Design review of the part built by this model. Coordinates are the model's own, in mm. Give positions to 0.01 mm unless a question says otherwise; leave off trailing zeros. Order: outer loops, then holes, each group sorted by start corner. A loop starts at its lowest first (then second) coordinate and runs counter-clockwise, first axis right, second up. Notation, with made-up numbers: M -23,21.5 L 14,21.5 A15 cw 14,47.5 Z; hole C 48.5,68.5 d7. An arc over 180 degrees is marked long. Answer as a JSON object with one key per item and string values.
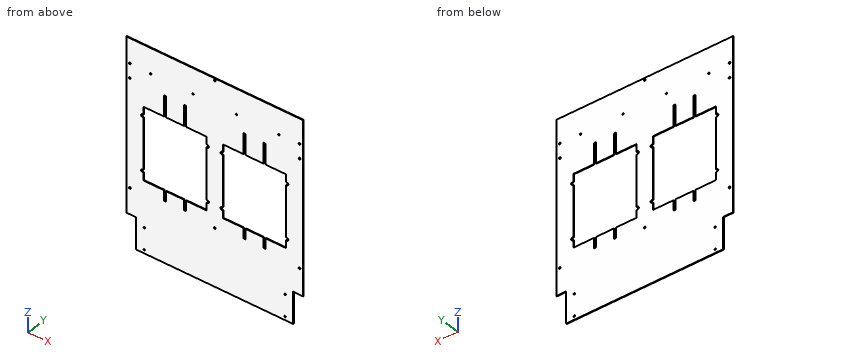
from build123d import *

# Parameters (mm, degrees)
F0_W     = 622.3
F0_H     = 717.55
F0_R     = 2.579688
F0_R_2   = 3.175
F1_DEPTH = 1.27
F2_W     = 34.925
F2_H     = 111.125
F2_W_2   = 6.35
F2_H_2   = 73.025
F2_H_3   = 36.5125
F2_R     = 2.579688
F3_DEPTH = 2.541


with BuildPart() as f1:
    # F0 (on Front) → F1 (new body, symmetric)
    with BuildSketch(Plane.XZ):
        Rectangle(F0_W, F0_H)
        with Locations((-247.65, -346.075)):
            Circle(F0_R, mode=Mode.SUBTRACT)
        with Locations((-247.65, -269.875)):
            Circle(F0_R, mode=Mode.SUBTRACT)
        with Locations((-298.45, -156.718)):
            Circle(F0_R_2, mode=Mode.SUBTRACT)
        with Locations((247.65, -346.075)):
            Circle(F0_R, mode=Mode.SUBTRACT)
        with Locations((247.65, -269.875)):
            Circle(F0_R, mode=Mode.SUBTRACT)
        with Locations((0, -156.718)):
            Circle(F0_R_2, mode=Mode.SUBTRACT)
        with Locations((298.45, -156.718)):
            Circle(F0_R_2, mode=Mode.SUBTRACT)
        with BuildLine():
            Line((-250.825, 117.856), (-250.825, 144.78))
            Line((-250.825, 144.78), (-28.575, 144.78))
            Line((-28.575, 144.78), (-28.575, 117.856))
            Line((-28.575, 117.856), (-25.4, 117.856))
            ThreePointArc((-25.4, 117.856), (-20.574, 113.03), (-25.4, 108.204))
            Line((-25.4, 108.204), (-28.575, 108.204))
            Line((-28.575, 108.204), (-28.575, -72.644))
            Line((-28.575, -72.644), (-25.4, -72.644))
            ThreePointArc((-25.4, -72.644), (-20.574, -77.47), (-25.4, -82.296))
            Line((-25.4, -82.296), (-28.575, -82.296))
            Line((-28.575, -82.296), (-28.575, -109.22))
            Line((-28.575, -109.22), (-250.825, -109.22))
            Line((-250.825, -109.22), (-250.825, -82.296))
            Line((-250.825, -82.296), (-254, -82.296))
            ThreePointArc((-254, -82.296), (-258.826, -77.47), (-254, -72.644))
            Line((-254, -72.644), (-250.825, -72.644))
            Line((-250.825, -72.644), (-250.825, 108.204))
            Line((-250.825, 108.204), (-254, 108.204))
            ThreePointArc((-254, 108.204), (-258.826, 113.03), (-254, 117.856))
            Line((-254, 117.856), (-250.825, 117.856))
        make_face(mode=Mode.SUBTRACT)
        with Locations((-298.45, 221.107)):
            Circle(F0_R_2, mode=Mode.SUBTRACT)
        with Locations((-298.45, 271.907)):
            Circle(F0_R_2, mode=Mode.SUBTRACT)
        with BuildLine():
            Line((28.575, -109.22), (28.575, -82.296))
            Line((28.575, -82.296), (25.4, -82.296))
            ThreePointArc((25.4, -82.296), (20.574, -77.47), (25.4, -72.644))
            Line((25.4, -72.644), (28.575, -72.644))
            Line((28.575, -72.644), (28.575, 108.204))
            Line((28.575, 108.204), (25.4, 108.204))
            ThreePointArc((25.4, 108.204), (20.574, 113.03), (25.4, 117.856))
            Line((25.4, 117.856), (28.575, 117.856))
            Line((28.575, 117.856), (28.575, 144.78))
            Line((28.575, 144.78), (250.825, 144.78))
            Line((250.825, 144.78), (250.825, 117.856))
            Line((250.825, 117.856), (254, 117.856))
            ThreePointArc((254, 117.856), (258.826, 113.03), (254, 108.204))
            Line((254, 108.204), (250.825, 108.204))
            Line((250.825, 108.204), (250.825, -72.644))
            Line((250.825, -72.644), (254, -72.644))
            ThreePointArc((254, -72.644), (258.826, -77.47), (254, -82.296))
            Line((254, -82.296), (250.825, -82.296))
            Line((250.825, -82.296), (250.825, -109.22))
            Line((250.825, -109.22), (28.575, -109.22))
        make_face(mode=Mode.SUBTRACT)
        with Locations((0, 351.282)):
            Circle(F0_R_2, mode=Mode.SUBTRACT)
        with Locations((298.45, 221.107)):
            Circle(F0_R_2, mode=Mode.SUBTRACT)
        with Locations((298.45, 271.907)):
            Circle(F0_R_2, mode=Mode.SUBTRACT)
    extrude(amount=F1_DEPTH, both=True)

    # F2 (on face) → F3 (cut, through all)
    with BuildSketch(Plane.XZ.offset(1.27)):
        with Locations((-293.6875, -303.2125)):
            Rectangle(F2_W, F2_H)
        with Locations((293.6875, -303.2125)):
            Rectangle(F2_W, F2_H)
        with Locations((-174.625, 181.2925)):
            Rectangle(F2_W_2, F2_H_2)
        with Locations((-104.775, 181.2925)):
            Rectangle(F2_W_2, F2_H_2)
        with Locations((-104.775, -127.47625)):
            Rectangle(F2_W_2, F2_H_3)
        with Locations((-174.625, -127.47625)):
            Rectangle(F2_W_2, F2_H_3)
        with Locations((104.775, 181.2925)):
            Rectangle(F2_W_2, F2_H_2)
        with Locations((174.625, -127.47625)):
            Rectangle(F2_W_2, F2_H_3)
        with Locations((174.625, 181.2925)):
            Rectangle(F2_W_2, F2_H_2)
        with Locations((104.775, -127.47625)):
            Rectangle(F2_W_2, F2_H_3)
        with Locations((225.425, 269.875)):
            Circle(F2_R)
        with Locations((-225.425, 269.875)):
            Circle(F2_R)
        with Locations((76.2, 269.875)):
            Circle(F2_R)
        with Locations((-76.2, 269.875)):
            Circle(F2_R)
    extrude(amount=-F3_DEPTH, mode=Mode.SUBTRACT)


solid = f1.part
(1) To check wall thickness, follow L1, parallel to Z at x = 298.45, y = 0 (3 decimals); L2, parallel to X at y = -1.05, z = 33 (3 decimals); L3, parallel to X at y = -0.55, z = -269.5 (3 decimals). State the ranges of each line that lie inside material, in increasing order. Write a range as from..to.
Checked values:
{"L1": "z = -247.65..-159.893, -153.543..217.932, 224.282..268.732, 275.082..358.775", "L2": "x = -311.15..-250.825, -28.575..28.575, 250.825..311.15", "L3": "x = -276.225..-250.202, -245.098..245.098, 250.202..276.225"}
(2) We need section B-B (x = 187). Write out the cut boundary in (y, z) (3 decimals), plus the area to 3 significant figures.
Checked values:
{"outline": "M -1.27,-358.775 L 1.27,-358.775 L 1.27,-109.22 L -1.27,-109.22 Z; M -1.27,144.78 L 1.27,144.78 L 1.27,358.775 L -1.27,358.775 Z", "area": "1,180 mm^2"}
(3) We need section A-A (z = -47). Write out the cut boundary in (x, y) (3 decimals).
Checked values:
{"outline": "M -311.15,-1.27 L -250.825,-1.27 L -250.825,1.27 L -311.15,1.27 Z; M -28.575,-1.27 L 28.575,-1.27 L 28.575,1.27 L -28.575,1.27 Z; M 250.825,-1.27 L 311.15,-1.27 L 311.15,1.27 L 250.825,1.27 Z"}
(4) We need section C-C (z = 194.5). Write out the cut boundary in (x, y).
Checked values:
{"outline": "M -311.15,-1.27 L -177.8,-1.27 L -177.8,1.27 L -311.15,1.27 Z; M -171.45,-1.27 L -107.95,-1.27 L -107.95,1.27 L -171.45,1.27 Z; M -101.6,-1.27 L 101.6,-1.27 L 101.6,1.27 L -101.6,1.27 Z; M 107.95,-1.27 L 171.45,-1.27 L 171.45,1.27 L 107.95,1.27 Z; M 177.8,-1.27 L 311.15,-1.27 L 311.15,1.27 L 177.8,1.27 Z"}
(5) We need section D-D (y = 0.6). Count the separate pieces of the cut face and the enclosed holes in it, plus the area to 3 significant figures.
Checked values:
{"separate pieces": "1", "enclosed holes": "18", "area": "322,000 mm^2"}
